Check sheet for the modelled part. Datum: model origin and axes. Units: mm. A direction names the side the tool comes from. Round coordinates to 2 decimals unless told otherwise and drop trailing zeros. Write each loop counter-clockwise with the first axis right and the second up, starting at its lowest first coordinate (ties: lowest second). Pieces come first, ordered by that corner, then holes. Notation, with made-up numbers: (41.25, -9.75) -> (89.25, -9.75) arc R23 ccw to (89.25, 17.25) -> close; hole circle Ø2 at (66.5, -1). An arc over 180 degrees is marked (long way). One line per item, written item: value.
from build123d import *

# Parameters (mm, degrees)
SKETCH1_R           = 20
BOSS_EXTRUDE1_DEPTH = 5
SKETCH2_R           = 11.5
SKETCH2_R_2         = 10.5
BOSS_EXTRUDE2_DEPTH = 70
SKETCH3_R           = 2.625
CUT_EXTRUDE1_DEPTH  = 81.156097709
CHAMFER1_SIZE       = 1.5
CHAMFER1_SIZE_2     = 4.121216129


with BuildPart() as part:
    # Sketch1 → Boss-Extrude1 (new body)
    with BuildSketch(Plane(origin=(0, 0, 0), x_dir=(1, 0, 0), z_dir=(0, 1, 0))):
        with Locations(Location((0, 0, 0), (0, 0, 270))):
            Circle(SKETCH1_R)
    extrude(amount=BOSS_EXTRUDE1_DEPTH)

    # Sketch2 → Boss-Extrude2 (add)
    with BuildSketch(Plane(origin=(0, 5, 0), x_dir=(1, 0, 0), z_dir=(0, 1, 0))):
        with Locations(Location((0, 0, 0), (0, 0, 270))):
            Circle(SKETCH2_R)
        with Locations(Location((0, 0, 0), (0, 0, 270))):
            Circle(SKETCH2_R_2, mode=Mode.SUBTRACT)
    extrude(amount=BOSS_EXTRUDE2_DEPTH)

    # Sketch3 → Cut-Extrude1 (cut, through all)
    with BuildSketch(Plane.XY):
        with Locations(Location((0, 35, 0), (0, 0, 180))):
            Circle(SKETCH3_R)
    extrude(amount=CUT_EXTRUDE1_DEPTH, mode=Mode.SUBTRACT)

    # Chamfer1
    # the kernel refuses this chamfer: 4.121216129, 1.5 mm, written as the material it takes off along each edge
    with BuildSketch(Plane(origin=(0, 75, 0), x_dir=(0, 0, 1), z_dir=(-1, 0, 0))) as chamfer1_piece_1:
        Polygon((10.5 + CHAMFER1_SIZE, 0), (10.5, -CHAMFER1_SIZE_2), (10.5, 0), align=None)
    revolve(axis=Axis((0, 75, 0), (0, 1, 0)), mode=Mode.SUBTRACT)


solid = part.part
Item 1: Sectioned sample at D-D on z = -16. Enter the section's corners in (x, y).
Answer:
outline: (-12, 0) -> (12, 0) -> (12, 5) -> (-12, 5) -> close
Item 2: Thickness scan on line 1 (X direction, y = 35, z = 0); line 2 (Y direction, x = -2, z = 3); line 3 (X direction, y = 8.5, z = 7). Record the ranges inside material, lowest first.
Answer:
line 1: x = -11.5 to -10.5, 10.5 to 11.5
line 2: y = 0 to 5
line 3: x = -9.12 to -7.83, 7.83 to 9.12
Item 3: Sectioned sample at B-B on z = 0. Enter the section's corners in (x, y), and give its area (3 significant figures).
Answer:
outline: (-20, 0) -> (20, 0) -> (20, 5) -> (11.5, 5) -> (11.5, 73.63) -> (10.5, 70.88) -> (10.5, 5) -> (-10.5, 5) -> (-10.5, 70.88) -> (-11.5, 73.63) -> (-11.5, 5) -> (-20, 5) -> close
area: 335 mm^2
Item 4: Mould release check, pull along Z, two halves, no side actions. Record for faces 4 (the flat face through (0, 5, 0)), 5 (the cylindrical face through (9.7, 38.83, 6.18)), 6 (the flat face through (0, 0, 0)): pulls with the +Z half, pulls with the -Z half, needs draft (parallel to the pull), parting line crosses it, or undercut.
Answer:
face 4: undercut
face 5: parting line crosses it
face 6: needs draft
Item 5: Depth check by flat-ended pin: P1, Ø1.5, axis at x = -1.5, z = 1.5, coming from the +Y side; P2, Ø12, axis at x = -15, y = 23.5, coming from the +Z side; P3, Ø8, axis at x = -12.5, y = 19, coming from the +Z side. Enter the tip coordinate at first touch or a pass-through.
Answer:
P1: stops at y = 5
P2: stops at z = 7.16
P3: stops at z = 7.75
Item 6: Tool access check on faces 1 (the cylindrical face through (-19.524, 2.465, -4.336)), 2 (the cylindrical face through (0.569, 37.563, 10.824)), 3 (the flat face through (-9, 5, 9)). Record the directions out of +Z, -Z, +X, -X, +Y, -Y that give a thin tool (end or side, any length) a straight path to the whole face; none if there is none.
Answer:
face 1: +Y, -Y
face 2: +Z
face 3: +Y
Item 7: Sectioned sample at A-A on x = 0. Enter the section's corners in (y, z) (3 decimals).
Answer:
outline: (0, -20) -> (5, -20) -> (5, -11.5) -> (73.626, -11.5) -> (70.879, -10.5) -> (5, -10.5) -> (5, 10.5) -> (32.375, 10.5) -> (32.375, 11.5) -> (5, 11.5) -> (5, 20) -> (0, 20) -> close; (37.625, 10.5) -> (70.879, 10.5) -> (73.626, 11.5) -> (37.625, 11.5) -> close
Item 8: Sectioned sample at C-C on y = 21. Enter the section's corners in (x, z).
Answer:
outline: circle Ø23 at (0, 0); hole circle Ø21 at (0, 0)
